Check sheet for the modelled part. Datum: model origin and axes. Units: mm. A direction names the side the tool comes from. Coordinates: 2 decimals unless noted, no trailing zeros. Order: outer loops, then holes, each group sorted by start corner. A loop starts at its lowest first (then second) coordinate and runs counter-clockwise, first axis right, second up.
from build123d import *

# Parameters (mm, degrees)
SKETCH_1_W          = 88.07644651
SKETCH_1_H          = 60
EXTRUDE_1_DEPTH     = 5
SKETCH_3_W          = 32.5
SKETCH_3_H          = 3
EXTRUDE_2_DEPTH     = 9.5
SKETCH_4_R          = 2.4
CUT_EXTRUDE_2_DEPTH = 100
SKETCH_5_W          = 32.5
SKETCH_5_H          = 34
EXTRUDE_3_DEPTH     = 2
SKETCH_6_R          = 2
CUT_EXTRUDE_3_DEPTH = 10


with BuildPart() as part:
    # 草图1 → 凸台-拉伸1 (new body)
    with BuildSketch(Plane.XY):
        with Locations((-26.142212211, -6.928181841)):
            Rectangle(SKETCH_1_W, SKETCH_1_H)
    extrude(amount=EXTRUDE_1_DEPTH)

    # 草图3 → 凸台-拉伸2 (add)
    with BuildSketch(Plane(origin=(0, 0, 0), x_dir=(-1, 0, 0), z_dir=(0, 0, -1))):
        with Locations((-1.646011044, 11.571818159)):
            Rectangle(SKETCH_3_W, SKETCH_3_H)
        with Locations((53.930435466, 11.571818159)):
            Rectangle(SKETCH_3_W, SKETCH_3_H)
        with Locations((-1.646011044, -25.428181841)):
            Rectangle(SKETCH_3_W, SKETCH_3_H)
        with Locations((53.930435466, -25.428181841)):
            Rectangle(SKETCH_3_W, SKETCH_3_H)
    extrude(amount=EXTRUDE_2_DEPTH)

    # 草图4 → 切除-拉伸2 (cut)
    with BuildSketch(Plane(origin=(0, -26.928181841, 0), x_dir=(-1, 0, 0), z_dir=(0, -1, 0))):
        with Locations(Location((-12.646011044, 5.25, 0), (0, 0, 90))):
            Circle(SKETCH_4_R)
        with Locations(Location((9.353988956, 5.25, 0), (0, 0, 90))):
            Circle(SKETCH_4_R)
        with Locations(Location((42.930435466, 5.25, 0), (0, 0, 90))):
            Circle(SKETCH_4_R)
        with Locations(Location((64.930435466, 5.25, 0), (0, 0, 90))):
            Circle(SKETCH_4_R)
    extrude(amount=-CUT_EXTRUDE_2_DEPTH, mode=Mode.SUBTRACT)

    # 草图5 → 凸台-拉伸3 (add)
    with BuildSketch(Plane(origin=(0, 0, 0), x_dir=(-1, 0, 0), z_dir=(0, 0, -1))):
        with Locations((-1.646011044, -6.928181841)):
            Rectangle(SKETCH_5_W, SKETCH_5_H)
        with Locations((53.930435466, -6.928181841)):
            Rectangle(SKETCH_5_W, SKETCH_5_H)
    extrude(amount=EXTRUDE_3_DEPTH)

    # 草图6 → 切除-拉伸3 (cut)
    with BuildSketch(Plane(origin=(0, 0, 0), x_dir=(-1, 0, 0), z_dir=(0, 0, -1))):
        with Locations((-12.896011044, 18.071818159)):
            Circle(SKETCH_6_R)
        with Locations((-12.896011044, -31.928181841)):
            Circle(SKETCH_6_R)
        with Locations((7.103988956, 18.071818159)):
            Circle(SKETCH_6_R)
        with Locations((7.103988956, -31.928181841)):
            Circle(SKETCH_6_R)
        with Locations((65.180435466, 18.071818159)):
            Circle(SKETCH_6_R)
        with Locations((65.180435466, -31.928181841)):
            Circle(SKETCH_6_R)
        with Locations((45.180435466, 18.071818159)):
            Circle(SKETCH_6_R)
        with Locations((45.180435466, -31.928181841)):
            Circle(SKETCH_6_R)
    extrude(amount=-CUT_EXTRUDE_3_DEPTH, mode=Mode.SUBTRACT)


solid = part.part
(1) Cross-section at A-A (x = -13.5). Enter the section's corners in (y, z), and give its area (3 significant figures).
Filled in:
outline: (-36.93, 0) - (-26.93, 0) - (-26.93, -9.5) - (-23.93, -9.5) - (-23.93, -2) - (10.07, -2) - (10.07, -9.5) - (13.07, -9.5) - (13.07, 0) - (23.07, 0) - (23.07, 5) - (-36.93, 5) - close
area: 425 mm2
(2) Release check for a two-part mould opening along Z. For faces 1 (the flat face through (2, -7, -2)), 2 (the cylindrical face through (11.97, -33.7, 2.46)), 3 (the cylindrical face through (-11.48, 11.55, -6.36)) record: +Z half, -Z half, draft (parallel to the pull), parting line (faces both ways), or undercut.
Filled in:
face 1: -Z half
face 2: draft
face 3: undercut
(3) Cross-section at B-B (y = -12.5). Enter the section's corners in (x, z), and give its area (3 significant figures).
Filled in:
outline: (-70.18, -2) - (-37.68, -2) - (-37.68, 0) - (-14.6, 0) - (-14.6, -2) - (17.9, -2) - (17.9, 5) - (-70.18, 5) - close
area: 570 mm2
(4) Tool access check on faces 4 (the flat face through (-37.68, -7.2, -1.5)), 5 (the cylindrical face through (-67.06, 11.55, -6.36)), 6 (the flat face through (2, 13.072, -5)), 7 (the flat face through (-54, 10.072, -6)), 8 (the cylindrical face through (-43.593, -33.145, 2.465)). Record the directions out of +Z, -Z, +X, -X, +Y, -Y that give a thin tool (end or side, any length) a straight path to the whole face; none if there is none.
Filled in:
face 4: -Z, +Y, -Y
face 5: +Y, -Y
face 6: -Z, +X, -X, +Y
face 7: -Z, +X, -X
face 8: +Z, -Z
(5) Go/stop test with flat-tipped pins: P1, Ø8, axis at x = -1, z = -7, coming from the +Y side; P2, Ø3, axis at x = -42.93, z = -5.25, coming from the -Y side; P3, Ø2, axis at x = -50.5, z = -4, coming from the -Y side; P4, Ø10, axis at x = -51, y = 0, coming from the -Z side. Record where each tip stops, or that it passes through.
Filled in:
P1: stops at y = 13.07
P2: passes through
P3: stops at y = -26.93
P4: stops at z = -2
(6) Thickness scan on probe 1 along Y at (x, z) = (13, 2.5); probe 2 along X at (y, z) = (-26.3, -5.25); probe 3 along Y at (x, z) = (-8, -3). Record the ranges inside material, lowest first.
Filled in:
probe 1: y = -36.93 to -33.93, -29.93 to 16.07, 20.07 to 23.07
probe 2: x = -70.18 to -67.33, -62.53 to -45.33, -40.53 to -37.68, -14.6 to -11.75, -6.95 to 10.25, 15.05 to 17.9
probe 3: y = -26.93 to -23.93, 10.07 to 13.07
(7) Cross-section at C-C (z = 3.5). Count the separate pieces of the cut face and the enclosed holes in it, and give its area (3 significant figures).
Filled in:
separate pieces: 1
enclosed holes: 8
area: 5,180 mm2
